Model file for the job. Use its own axes, mm. Coordinates: 2 decimals unless noted, no trailing zeros. Order: outer loops, then holes, each group sorted by start corner. A loop starts at its lowest first (then second) coordinate and runs counter-clockwise, first axis right, second up. Notation, with made-up numbers: (-8, -17) -> (2, -17) arc R31 ccw to (2, 15) -> close; hole circle Ø4 at (84, 80.5). An arc over 180 degrees is marked (long way). Return JSON: item names as keys, results as strings. Group by question number.
1) Cut at B-B (z = 15.24). Write the cut outline in (x, y) (3 decimals).
2) Cut at A-A (x = -7). Write the cut outline in (y, z) (3 decimals), and give its area (3 significant figures).
3) Probe line 1 (Y direction, x = 9, z = 96.5) (3 decimals); line 2 (Z direction, x = -11.5, y = -1.75). List the from-to ranges inside material, lowest first.
4) Cut at C-C (y = 0). State how many separate pieces and enclosed holes the cut face has, and give its area (3 significant figures).
5) Flat gauge pin, fed straight in: pin 1 (6 mm diameter, centred on x = 0, z = 228.6, fed in from -Y). Where does the tip first touch, or does it go through?
6) Cut at D-D (z = 102). Write the cut outline in (x, y) (3 decimals), and give its area (3 significant figures).
from build123d import *

# Parameters (mm, degrees)
SKETCH2_W           = 25.4
SKETCH2_H           = 25.4
BOSS_EXTRUDE1_DEPTH = 279.4
SKETCH4_W           = 19.05
SKETCH4_H           = 19.05
CUT_EXTRUDE1_DEPTH  = 280.9766776
SKETCH5_R           = 3.2639
CUT_EXTRUDE2_DEPTH  = 281.839473721
SKETCH6_R           = 3.2639
CUT_EXTRUDE3_DEPTH  = 281.839473721
SKETCH7_R           = 3.2639
CUT_EXTRUDE4_DEPTH  = 281.839473721
SKETCH8_R           = 3.2639
CUT_EXTRUDE5_DEPTH  = 281.839473721


with BuildPart() as part:
    # Sketch2 → Boss-Extrude1 (new body)
    with BuildSketch(Plane.XY):
        Rectangle(SKETCH2_W, SKETCH2_H)
    extrude(amount=BOSS_EXTRUDE1_DEPTH)

    # Sketch4 → Cut-Extrude1 (cut, through all)
    with BuildSketch(Plane.XY):
        Rectangle(SKETCH4_W, SKETCH4_H)
    extrude(amount=CUT_EXTRUDE1_DEPTH, mode=Mode.SUBTRACT)

    # Sketch5 → Cut-Extrude2 (cut, through all)
    with BuildSketch(Plane(origin=(0, 12.7, 0), x_dir=(1, 0, 0), z_dir=(0, 1, 0))):
        with Locations(Location((0, -15.24, 0), (0, 0, 270))):
            Circle(SKETCH5_R)
    extrude(amount=-CUT_EXTRUDE2_DEPTH, mode=Mode.SUBTRACT)

    # Sketch6 → Cut-Extrude3 (cut, through all)
    with BuildSketch(Plane(origin=(0, 12.7, 0), x_dir=(1, 0, 0), z_dir=(0, 1, 0))):
        with Locations(Location((0, -228.6, 0), (0, 0, 270))):
            Circle(SKETCH6_R)
    extrude(amount=-CUT_EXTRUDE3_DEPTH, mode=Mode.SUBTRACT)

    # Sketch7 → Cut-Extrude4 (cut, through all)
    with BuildSketch(Plane.ZY.offset(12.7)):
        with Locations((15.24, 0)):
            Circle(SKETCH7_R)
    extrude(amount=-CUT_EXTRUDE4_DEPTH, mode=Mode.SUBTRACT)

    # Sketch8 → Cut-Extrude5 (cut, through all)
    with BuildSketch(Plane.ZY.offset(12.7)):
        with Locations((198.12, 0)):
            Circle(SKETCH8_R)
        with Locations((147.32, 0)):
            Circle(SKETCH8_R)
    extrude(amount=-CUT_EXTRUDE5_DEPTH, mode=Mode.SUBTRACT)


solid = part.part
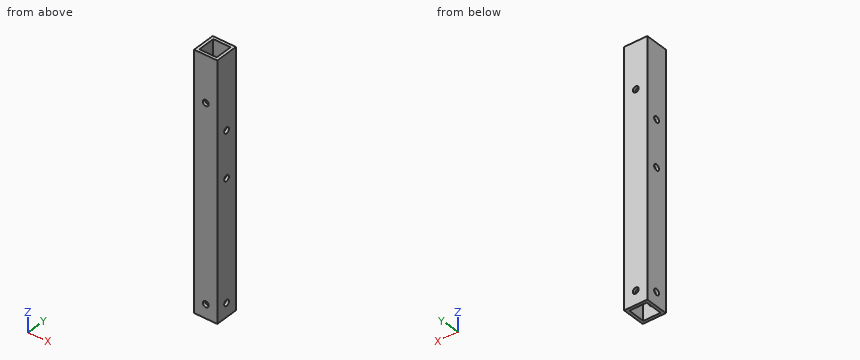
Answers below:
{
 "1": {"outline": "(-12.7, -12.7) -> (-3.264, -12.7) -> (-3.264, -9.525) -> (-9.525, -9.525) -> (-9.525, -3.264) -> (-12.7, -3.264) -> close; (-12.7, 3.264) -> (-9.525, 3.264) -> (-9.525, 9.525) -> (-3.264, 9.525) -> (-3.264, 12.7) -> (-12.7, 12.7) -> close; (3.264, -12.7) -> (12.7, -12.7) -> (12.7, -3.264) -> (9.525, -3.264) -> (9.525, -9.525) -> (3.264, -9.525) -> close; (3.264, 9.525) -> (9.525, 9.525) -> (9.525, 3.264) -> (12.7, 3.264) -> (12.7, 12.7) -> (3.264, 12.7) -> close"},
 "2": {"outline": "(-12.7, 0) -> (-9.525, 0) -> (-9.525, 279.4) -> (-12.7, 279.4) -> close; (9.525, 0) -> (12.7, 0) -> (12.7, 279.4) -> (9.525, 279.4) -> close", "area": "1,770 mm^2"},
 "3": {"line 1": "y = -12.7 to -9.525, 9.525 to 12.7", "line 2": "z = 0 to 12.48, 18 to 144.56, 150.08 to 195.36, 200.88 to 279.4"},
 "4": {"separate pieces": "8", "enclosed holes": "0", "area": "1,650 mm^2"},
 "5": {"pin 1": "passes through"},
 "6": {"outline": "(-12.7, -12.7) -> (12.7, -12.7) -> (12.7, 12.7) -> (-12.7, 12.7) -> close; hole (-9.525, -9.525) -> (9.525, -9.525) -> (9.525, 9.525) -> (-9.525, 9.525) -> close", "area": "282 mm^2"}
}
